Autodesk Inventor part; units mm, degrees
ref_plane "YZ Plane" through (0, 0, 0) normal (1, 0, 0) x (0, 1, 0)
ref_plane "XZ Plane" through (0, 0, 0) normal (0, 1, 0) x (-1, 0, 0)
ref_plane "XY Plane" through (0, 0, 0) normal (0, 0, 1) x (1, 0, 0)
sketch "Sketch1" plane through (0, 0, 0) normal (0, 0, 1) x (1, 0, 0)
  line L0 (0, 0) -> (3.1, 0) construction
  circle A0 centre (0, 0) radius 2.0286 construction
  line L1 (0, 0) -> (1.55, 2.6847) construction
  line L2 (0, 0) -> (-1.55, 2.6847) construction
  line L3 (0, 0) -> (-3.1, 0) construction
  line L4 (0, 0) -> (-1.55, -2.6847) construction
  line L5 (0, 0) -> (1.55, -2.6847) construction
  line L6 (-1.55, 2.6847) -> (1.55, 2.6847)
  line L7 (1.55, 2.6847) -> (3.1, 0)
  line L8 (3.1, 0) -> (1.55, -2.6847)
  line L9 (1.55, -2.6847) -> (-1.55, -2.6847)
  line L10 (-1.55, -2.6847) -> (-3.1, 0)
  line L11 (-3.1, 0) -> (-1.55, 2.6847)
  dimension "d0" = 3.1
  dimension "d3" = 360
extrude "Extrusion1" add sketch "Sketch1" along normal blind 115
sketch "Sketch2" plane through (-1.55, -2.6847, 0) normal (0, -1, 0) x (1, 0, 0)
  circle A0 centre (1.55, 5) radius 0.65
  line L0 (3.1, 0) -> (3.1, 115)
  line L1 (0, 0) -> (0, 115)
  line L2 (0, 0) -> (3.1, 0)
  circle A1 centre (1.55, 60) radius 0.65
  circle A2 centre (1.55, 57) radius 0.65
  point P0 (1.55, 0)
  point P1 (1.55, 0)
  dimension "d7" = 1.3
  dimension "d8" = 5
  dimension "d9" = 60
  dimension "d10" = 3
extrude "Extrusion2" cut sketch "Sketch2" against normal blind 10
properties part number "eje1_n"
The model under review builds one solid part; all positions refer to its coordinate system, in mm. Give positions to 0.01 mm unless a question says otherwise; leave off trailing zeros. Write each loop counter-clockwise with the first axis right and the second up, starting at its lowest first coordinate (ties: lowest second). Pieces come first, ordered by that corner, then holes. Notation, with made-up numbers: (26, -6) -> (61, -6) arc R11 cw to (61, 9) -> close; hole circle Ø7 at (28.25, -31). An arc over 180 degrees is marked (long way). Answer in a Markdown table with one row per item.
1) Clearance check with flat-ended pins moving along their axes: P1, Ø1, axis at x = 0, z = 60, coming from the +Y side; P2, Ø3, axis at y = 2, z = 22, coming from the +X side. State where each tip first meets the part, or that it passes through.
Worked answers:
| item | result |
|---|---|
| P1 | through |
| P2 | x = 2.81 |
2) For L1, parallel to Z at x = 0, y = -0.45; L2, parallel to X at y = 0.5, z = 57; L3, parallel to X at y = 1, z = 57, list the stretches that pass through material, from the lowest coordinate up. Write a range as [from, to].
Worked answers:
| item | result |
|---|---|
| L1 | [0, 4.35], [5.65, 56.35], [57.65, 59.35], [60.65, 115] |
| L2 | [-2.81, -0.65], [0.65, 2.81] |
| L3 | [-2.52, -0.65], [0.65, 2.52] |
3) Add section B-B on z = 31. State the section outline as (x, y) points.
Worked answers:
| item | result |
|---|---|
| outline | (-3.1, 0) -> (-1.55, -2.68) -> (1.55, -2.68) -> (3.1, 0) -> (1.55, 2.68) -> (-1.55, 2.68) -> close |
4) Add section A-A on y = 1.25. State the section outline as (x, z) points, plus the area to 3 significant figures.
Worked answers:
| item | result |
|---|---|
| outline | (-2.38, 0) -> (2.38, 0) -> (2.38, 115) -> (-2.38, 115) -> close; hole circle Ø1.3 at (0, 5); hole circle Ø1.3 at (0, 57); hole circle Ø1.3 at (0, 60) |
| area | 543 mm² |
